Source: CAD feature listing. Evaluate the final solid. Frame: model axes, mm. Coordinates: 2 decimals unless noted, no trailing zeros. Order: outer loops, then holes, each group sorted by start corner. A loop starts at its lowest first (then second) coordinate and runs counter-clockwise, first axis right, second up.
Autodesk Inventor part; units mm, degrees
ref_plane "YZ Plane" through (0, 0, 0) normal (1, 0, 0) x (0, 1, 0)
ref_plane "XZ Plane" through (0, 0, 0) normal (0, 1, 0) x (-1, 0, 0)
ref_plane "XY Plane" through (0, 0, 0) normal (0, 0, 1) x (1, 0, 0)
sketch "Sketch1" plane through (0, 0, 0) normal (0, 1, 0) x (-1, 0, 0)
  circle A0 centre (0, 0) radius 90 construction
  line L0 (-55, 71.239) -> (-55, -71.239) construction
  line L1 (-45, 75) -> (25, 75) construction
  line L2 (25, 75) -> (25, 60) construction
  line L3 (25, 60) -> (-45, 60) construction
  line L4 (-45, 60) -> (-45, 75) construction
  line L5 (-55, 0) -> (0, 0) construction
  circle A1 centre (0, 0) radius 90 construction
  line L6 (-45, -75) -> (25, -75) construction
  line L7 (25, -75) -> (25, -60) construction
  line L8 (25, -60) -> (-45, -60) construction
  line L9 (-45, -60) -> (-45, -75) construction
  line L10 (-10, 60) -> (-10, -60) construction
  dimension "d0" = 180
  dimension "d1" = 55
  dimension "d2" = 70
  dimension "d3" = 60
  dimension "d4" = 10
  dimension "d5" = 15
sketch "Sketch2" plane through (0, 0, 0) normal (0, 1, 0) x (-1, 0, 0)
  circle A0 centre (0, 0) radius 90
  line L0 (-55, -71.239) -> (-55, 71.239)
  dimension "d6" = 180
  dimension "d7" = 55
extrude "Extrusion1" add sketch "Sketch2" along normal blind 3 contours A0 L0 picked at (-6.6667, 0)
sketch "Sketch3" plane through (0, 3, 0) normal (0, 1, 0) x (1, 0, 0)
  line L0 (-25, -60) -> (45, -60) construction
  line L1 (45, -60) -> (45, -75) construction
  line L2 (-25, -75) -> (-25, -60) construction
  line L3 (45, -75) -> (-25, -75) construction
  line L4 (45, -60) -> (-25, -60)
  line L5 (-25, -60) -> (-25, -75)
  line L6 (-25, -75) -> (45, -75)
  line L7 (45, -75) -> (45, -60)
  point P0 (0, 0)
extrude "Extrusion2" cut sketch "Sketch3" against normal blind 3
mirror "Mirror1" about plane through (0, 0, 0) normal (0, 0, 1) of "Extrusion2"
sketch "Sketch4" plane through (0, 3, 0) normal (0, 1, 0) x (1, 0, 0)
  line L0 (10, -60) -> (10, 60)
  line L1 (22.5, -5) -> (-2.5, -5) construction
  line L2 (-2.5, -5) -> (-2.5, -57) construction
  line L3 (-2.5, -57) -> (22.5, -57) construction
  line L4 (22.5, -57) -> (22.5, -5) construction
  line L5 (22.5, -5) -> (-2.5, -57) construction
  line L6 (-2.5, -5) -> (22.5, -57) construction
  line L7 (-25, -60) -> (45, -60) construction
  line L8 (45, 60) -> (-25, 60) construction
  line L9 (45, -60) -> (-25, -60)
  line L10 (-2.5, -60) -> (-12.5, -60)
  line L11 (-12.5, -60) -> (-12.5, -57)
  line L12 (-12.5, -57) -> (-2.5, -57)
  line L13 (-2.5, -57) -> (-2.5, -60)
  line L14 (22.5, -57) -> (32.5, -57)
  line L15 (32.5, -57) -> (32.5, -60)
  line L16 (32.5, -60) -> (22.5, -60)
  line L17 (22.5, -60) -> (22.5, -57)
  line L18 (-2.5, -37) -> (-5.5, -37)
  line L19 (-5.5, -37) -> (-5.5, -27)
  line L20 (-5.5, -27) -> (-2.5, -27)
  line L21 (-2.5, -27) -> (-2.5, -37)
  line L22 (22.5, -37) -> (25.5, -37)
  line L23 (25.5, -37) -> (25.5, -27)
  line L24 (25.5, -27) -> (22.5, -27)
  line L25 (22.5, -27) -> (22.5, -37)
  point P0 (0, 0)
  point P1 (10, -31)
  dimension "d12" = 25
  dimension "d13" = 52
  dimension "d14" = 3
  dimension "d15" = 10
  dimension "d16" = 10
  dimension "d17" = 3
  dimension "d18" = 10
  dimension "d19" = 20
  dimension "d20" = 3
  dimension "d21" = 10
extrude "Extrusion3" cut sketch "Sketch4" against normal blind 3
sketch "Sketch5" plane through (0, 3, 0) normal (0, 1, 0) x (1, 0, 0)
  line L0 (55, -71.239) -> (55, 71.239)
  line L1 (55, -65) -> (52, -65)
  line L2 (52, -65) -> (52, -45)
  line L3 (52, -45) -> (55, -45)
  line L4 (55, -45) -> (55, -65)
  line L5 (55, -25) -> (52, -25)
  line L6 (52, -25) -> (52, -5)
  line L7 (52, -5) -> (55, -5)
  line L8 (55, -5) -> (55, -25)
  point P0 (0, 0)
  dimension "d24" = 3
  dimension "d25" = 20
  dimension "d26" = 20
  dimension "d27" = 20
  dimension "d28" = 5
extrude "Extrusion4" cut sketch "Sketch5" against normal blind 3
mirror "Mirror2" about plane through (0, 0, 0) normal (0, 0, 1) of "Extrusion3", "Extrusion4"
properties part number "BasePlate"
1. Section query C-C, the plane z = 63. Output: boundary loops of the cut face in (x, y), plus the area to 3 significant figures.
2. Contact query for flat-ended pins moving along their axis: P1, Ø1.5, axis at y = 1, z = -58.5, coming from the -X side; P2, Ø1.5, axis at x = 53, y = 2, coming from the -Z side; P3, Ø1.5, axis at y = 2, z = 58, coming from the +X side; P4, Ø8, axis at x = 1.5, z = -70.5, coming from the +Y side. Output: stop coordinate, or through.
3. Section query D-D, the plane y = 2.45. Count the separate pieces of the cut face and the enclosed holes in it, plus the area to 3 significant figures.
4. Section query A-A, the plane x = 0. Output: boundary loops of the cut face in (y, z), plus the area to 3 significant figures.
5. Material intervals for line 1 along X through (y, z) = (1.45, -32.5); line 2 along Z through (x, y) = (-20, 2.4); line 3 along X through (y, z) = (2.6, -36), sorted ascending.
6. Section query B-B, the plane z = -34.5. Output: boundary loops of the cut face in (x, y), plus the area to 3 significant figures.
Answer key:
1. outline: (-64.27, 0) - (-25, 0) - (-25, 3) - (-64.27, 3) - close; (45, 0) - (52, 0) - (52, 3) - (45, 3) - close
1. area: 139 mm2
2. P1: stops at x = -69.03
2. P2: stops at z = -73.28
2. P3: stops at x = 52
2. P4: passes through
3. separate pieces: 1
3. enclosed holes: 6
3. area: 19,400 mm2
4. outline: (0, -90) - (3, -90) - (3, -75) - (0, -75) - close; (0, -60) - (3, -60) - (3, 60) - (0, 60) - close; (0, 75) - (3, 75) - (3, 90) - (0, 90) - close
4. area: 450 mm2
5. line 1: x = -83.93 to -5.5, -2.5 to 22.5, 25.5 to 55
5. line 2: z = -87.75 to -75, -60 to 60, 75 to 87.75
5. line 3: x = -82.49 to -5.5, -2.5 to 22.5, 25.5 to 55
6. outline: (-83.12, 0) - (-5.5, 0) - (-5.5, 3) - (-83.12, 3) - close; (-2.5, 0) - (22.5, 0) - (22.5, 3) - (-2.5, 3) - close; (25.5, 0) - (55, 0) - (55, 3) - (25.5, 3) - close
6. area: 396 mm2
